Work out the finished part from the listing and answer in its coordinate system (mm). Coordinates: 2 decimals unless noted, no trailing zeros. Answer as CSV lines item,"result".
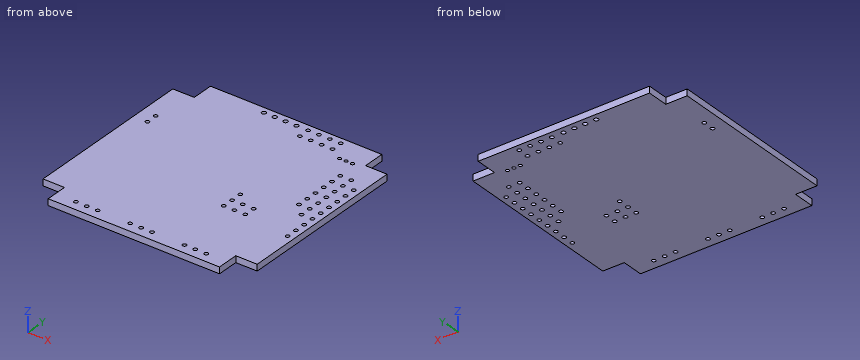
```python
from build123d import *

# Parameters (mm, degrees)
SKETCH_3_R      = 0.4499991
SKETCH_3_R_2    = 0.3999992
SKETCH_3_R_3    = 0.499999
EXTRUDE_1_DEPTH = 1.5


with BuildPart() as part:
    # Эскиз3 → Бобышка-Вытянуть1 (new body)
    with BuildSketch(Plane.XY):
        Polygon((24.081237265, -17.758826004), (24.081237265, 22.241173056), (19.081237265, 22.241173056), (19.081237265, 27.241173056), (-20.918761795, 27.241173056), (-20.918761795, 22.241173056), (-25.918761795, 22.241173056), (-25.918761795, -17.758826004), (-20.918761795, -17.758826004), (-20.918761795, -22.758826004), (19.081237265, -22.758826004), (19.081237265, -17.758826004), align=None)
        with Locations((22.581258045, 1.241166636)):
            Circle(SKETCH_3_R, mode=Mode.SUBTRACT)
        with Locations((22.581258045, 3.791174236)):
            Circle(SKETCH_3_R, mode=Mode.SUBTRACT)
        with Locations((22.581258045, 6.341181836)):
            Circle(SKETCH_3_R, mode=Mode.SUBTRACT)
        with Locations((22.581258045, 8.891189436)):
            Circle(SKETCH_3_R, mode=Mode.SUBTRACT)
        with Locations((22.581258045, 11.441197036)):
            Circle(SKETCH_3_R, mode=Mode.SUBTRACT)
        with Locations((22.581258045, 13.991204636)):
            Circle(SKETCH_3_R, mode=Mode.SUBTRACT)
        with Locations((17.501258045, 3.791174236)):
            Circle(SKETCH_3_R, mode=Mode.SUBTRACT)
        with Locations((17.501258045, 6.341181836)):
            Circle(SKETCH_3_R, mode=Mode.SUBTRACT)
        with Locations((17.501258045, 8.891189436)):
            Circle(SKETCH_3_R, mode=Mode.SUBTRACT)
        with Locations((17.501258045, 11.441197036)):
            Circle(SKETCH_3_R, mode=Mode.SUBTRACT)
        with Locations((17.501258045, 13.991204636)):
            Circle(SKETCH_3_R, mode=Mode.SUBTRACT)
        with Locations((17.501258045, 16.541212236)):
            Circle(SKETCH_3_R, mode=Mode.SUBTRACT)
        with Locations((20.041258045, 16.541212236)):
            Circle(SKETCH_3_R, mode=Mode.SUBTRACT)
        with Locations((20.041258045, 13.991204636)):
            Circle(SKETCH_3_R, mode=Mode.SUBTRACT)
        with Locations((20.041258045, 11.441197036)):
            Circle(SKETCH_3_R, mode=Mode.SUBTRACT)
        with Locations((20.041258045, 8.891189436)):
            Circle(SKETCH_3_R, mode=Mode.SUBTRACT)
        with Locations((20.041258045, 6.341181836)):
            Circle(SKETCH_3_R, mode=Mode.SUBTRACT)
        with Locations((20.041258045, 3.791174236)):
            Circle(SKETCH_3_R, mode=Mode.SUBTRACT)
        with Locations((20.041258045, 1.241166636)):
            Circle(SKETCH_3_R, mode=Mode.SUBTRACT)
        with Locations((22.581235185, -6.388825724)):
            Circle(SKETCH_3_R, mode=Mode.SUBTRACT)
        with Locations((22.581235185, -3.848825724)):
            Circle(SKETCH_3_R, mode=Mode.SUBTRACT)
        with Locations((22.581235185, -1.308825724)):
            Circle(SKETCH_3_R, mode=Mode.SUBTRACT)
        with Locations((3.011236225, 25.741170976)):
            Circle(SKETCH_3_R, mode=Mode.SUBTRACT)
        with Locations((5.551236225, 23.201170976)):
            Circle(SKETCH_3_R, mode=Mode.SUBTRACT)
        with Locations((5.551236225, 25.741170976)):
            Circle(SKETCH_3_R, mode=Mode.SUBTRACT)
        with Locations((8.091236225, 23.201170976)):
            Circle(SKETCH_3_R, mode=Mode.SUBTRACT)
        with Locations((8.091236225, 25.741170976)):
            Circle(SKETCH_3_R, mode=Mode.SUBTRACT)
        with Locations((10.631236225, 25.741170976)):
            Circle(SKETCH_3_R, mode=Mode.SUBTRACT)
        with Locations((10.631236225, 23.201170976)):
            Circle(SKETCH_3_R, mode=Mode.SUBTRACT)
        with Locations((13.706236425, 21.341172156)):
            Circle(SKETCH_3_R_2, mode=Mode.SUBTRACT)
        with Locations((15.206235965, 21.341172156)):
            Circle(SKETCH_3_R_2, mode=Mode.SUBTRACT)
        with Locations((16.706235505, 21.341172156)):
            Circle(SKETCH_3_R_2, mode=Mode.SUBTRACT)
        with Locations((6.656270845, 0.041156336)):
            Circle(SKETCH_3_R, mode=Mode.SUBTRACT)
        with Locations((6.656270845, -5.038843664)):
            Circle(SKETCH_3_R, mode=Mode.SUBTRACT)
        with Locations((6.656270845, -2.498843664)):
            Circle(SKETCH_3_R, mode=Mode.SUBTRACT)
        with Locations((9.131325585, -2.498843664)):
            Circle(SKETCH_3_R, mode=Mode.SUBTRACT)
        with Locations((9.131325585, -5.038843664)):
            Circle(SKETCH_3_R, mode=Mode.SUBTRACT)
        with Locations((11.681361125, -2.498843664)):
            Circle(SKETCH_3_R, mode=Mode.SUBTRACT)
        with Locations((14.261284845, -20.508802564)):
            Circle(SKETCH_3_R, mode=Mode.SUBTRACT)
        with Locations((11.721284845, -20.508802564)):
            Circle(SKETCH_3_R, mode=Mode.SUBTRACT)
        with Locations((9.181284845, -20.508802564)):
            Circle(SKETCH_3_R, mode=Mode.SUBTRACT)
        with Locations((1.598775245, -20.508802564)):
            Circle(SKETCH_3_R, mode=Mode.SUBTRACT)
        with Locations((-0.941224755, -20.508802564)):
            Circle(SKETCH_3_R, mode=Mode.SUBTRACT)
        with Locations((-3.481224755, -20.508802564)):
            Circle(SKETCH_3_R, mode=Mode.SUBTRACT)
        with Locations((-11.063734355, -20.508802564)):
            Circle(SKETCH_3_R, mode=Mode.SUBTRACT)
        with Locations((-13.603734355, -20.508802564)):
            Circle(SKETCH_3_R, mode=Mode.SUBTRACT)
        with Locations((-16.143734355, -20.508802564)):
            Circle(SKETCH_3_R, mode=Mode.SUBTRACT)
        with Locations((-22.668758135, 10.141171696)):
            Circle(SKETCH_3_R, mode=Mode.SUBTRACT)
        with Locations((-22.668758135, 12.681171696)):
            Circle(SKETCH_3_R, mode=Mode.SUBTRACT)
        with Locations((-7.333782455, 25.756172216)):
            Circle(SKETCH_3_R_3, mode=Mode.SUBTRACT)
        with Locations((-4.793782455, 25.756172216)):
            Circle(SKETCH_3_R_3, mode=Mode.SUBTRACT)
        with Locations((-2.253782455, 25.756172216)):
            Circle(SKETCH_3_R_3, mode=Mode.SUBTRACT)
        with Locations((0.286217545, 25.756172216)):
            Circle(SKETCH_3_R_3, mode=Mode.SUBTRACT)
        with Locations((3.011236225, 23.201170976)):
            Circle(SKETCH_3_R, mode=Mode.SUBTRACT)
        with Locations((11.681361125, -5.038843664)):
            Circle(SKETCH_3_R, mode=Mode.SUBTRACT)
    extrude(amount=EXTRUDE_1_DEPTH)


solid = part.part
```
(1) A cutting plane is placed at A-A, the plane z = 0.75. Count the separate pieces of the cut face and the enclosed holes in it, and give its area (3 significant figures).
Computed values:
separate pieces,"1"
enclosed holes,"55"
area,"2,360 mm2"
(2) Flat-ended cylindrical pins translate along their axes: pin 1 Ø0.8 at (y, z) = (25, 0.5) entering from -X; pin 2 Ø0.8 at (x, z) = (-22.5, 0.5) entering from +Y. Find the tip coordinate at first contact, or state that the pin passes through.
Computed values:
pin 1,"x = -20.92"
pin 2,"y = 22.24"
(3) Consider line 1 along X through (y, z) = (0, 0.2); line 2 along X through (y, z) = (4, 0.7); line 3 along Y through (x, z) = (10.5, 0.5). Determine where each line is inside the solid, lowest interval first.
Computed values:
line 1,"-25.92 to 6.21, 7.1 to 24.08"
line 2,"-25.92 to 17.1, 17.9 to 19.64, 20.44 to 22.18, 22.98 to 24.08"
line 3,"-22.76 to 22.77, 23.63 to 25.31, 26.17 to 27.24"
